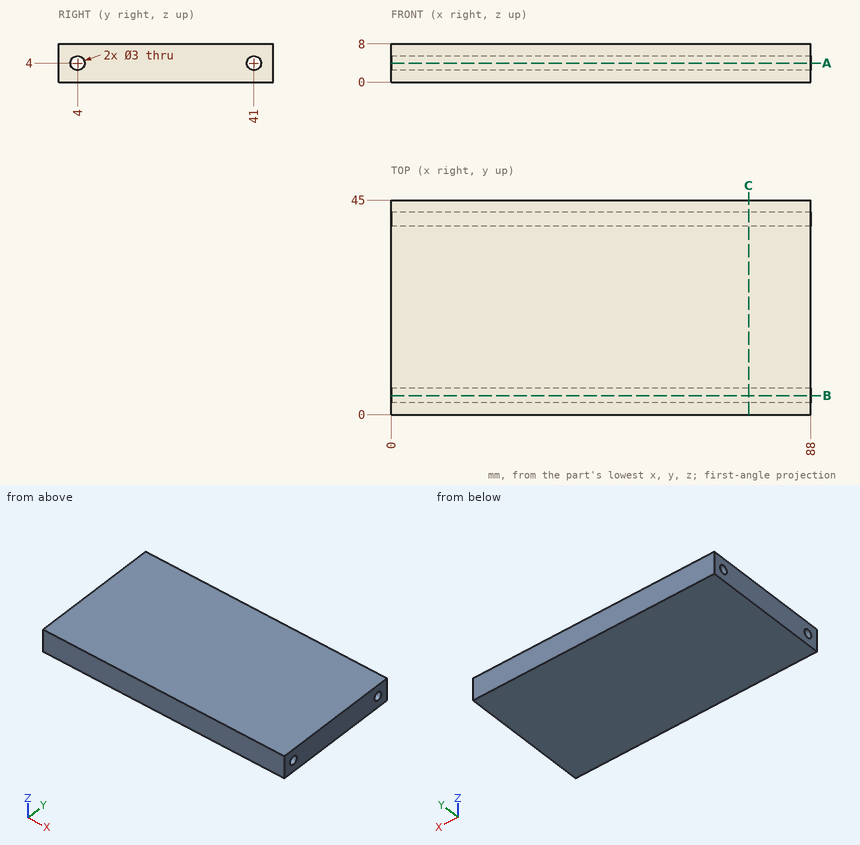
Check sheet for the drawn part. Datum: minimum x, y, z corner. Units: mm. Round coordinates to 2 decimals unless told otherwise and drop trailing zeros. Write each loop counter-clockwise with the first axis right and the second up, starting at its lowest first coordinate (ties: lowest second). Pieces come first, ordered by that corner, then holes. Notation, with made-up numbers: (-5.5, 45) - (14.5, 45) arc R25 cw to (14.5, 79) - close; hole circle Ø4 at (49, -16). An arc over 180 degrees is marked (long way). Return JSON: item names as keys, results as strings.
Q1. Cross-section at B-B (y = 4). Record the boundary of the cut face in (x, z).
Returned:
{"outline": "(0, 0) - (88, 0) - (88, 2.5) - (0, 2.5) - close; (0, 5.5) - (88, 5.5) - (88, 8) - (0, 8) - close"}
Q2. Depth check by flat-ended pin: P1, Ø1.5, axis at x = 17, z = 3.5, coming from the -Y side. Enter the tip coordinate at first touch or a pass-through.
Returned:
{"P1": "stops at y = 0"}
Q3. Cross-section at C-C (x = 75). Record the boundary of the cut face in (y, z).
Returned:
{"outline": "(0, 0) - (45, 0) - (45, 8) - (0, 8) - close; hole circle Ø3 at (4, 4); hole circle Ø3 at (41, 4)"}
Q4. Scan lines: L1, parallel to Y at x = 26, z = 4; L2, parallel to Y at x = 65, z = 4.5; L3, parallel to Z at x = 11.5, y = 42. Record each from-to range of solid material in increasing order. Write a range as from..to.
Returned:
{"L1": "y = 0..2.5, 5.5..39.5, 42.5..45", "L2": "y = 0..2.59, 5.41..39.59, 42.41..45", "L3": "z = 0..2.88, 5.12..8"}
Q5. Cross-section at A-A (z = 4). Record the boundary of the cut face in (x, y).
Returned:
{"outline": "(0, 0) - (88, 0) - (88, 2.5) - (0, 2.5) - close; (0, 5.5) - (88, 5.5) - (88, 39.5) - (0, 39.5) - close; (0, 42.5) - (88, 42.5) - (88, 45) - (0, 45) - close"}
